Work out the finished part from the listing and answer in its coordinate system (mm). Face numbers are marked on the shaded views. A direction names the side the tool comes from. Give positions to 0.01 mm unless a question says otherwise; leave off trailing zeros. Order: outer loops, then holes, each group sorted by start corner. A loop starts at its lowest first (then second) coordinate and runs counter-clockwise, first axis right, second up.
```python
from build123d import *

# Parameters (mm, degrees)
EXTRUDE_1_DEPTH          = 2.5
SKETCH_5_R               = 0.6
CUT_EXTRUDE_1_DEPTH      = 19.036421485
CUT_EXTRUDE_START        = -2
SKETCH_5_3_R             = 1
CUT_EXTRUDE_2_DEPTH      = 1
REVOLVE_1_ANGLE          = 1
SKETCH_9_R               = 0.6
CUT_EXTRUDE_3_DEPTH      = 41.426698916
SKETCH_9_3_R             = 1
CUT_EXTRUDE_4_DEPTH      = 1
SKETCH_10_W              = 73.33326834
SKETCH_10_H              = 28.500223869
CUT_EXTRUDE_5_DEPTH      = 41.528606999
CUT_EXTRUDE_8_DEPTH      = 41.426698916
CUT_EXTRUDE_8_DEPTH_BACK = 41.426698916


with BuildPart() as part:
    # 草图4 → 凸台-拉伸1 (new body)
    with BuildSketch(Plane.XY):
        Polygon((8.5, -1.5), (17.75, -1.5), (17.75, -3.5), (-4.5, -3.5), (-4.5, -1.5), (-0.5, 0), (0, 0), (0, -1.5), (4, -1.5), (4, 0), (4.5, 0), align=None)
    extrude(amount=EXTRUDE_1_DEPTH)

    # 草图5 → 切除-拉伸1 (cut, through all)
    with BuildSketch(Plane(origin=(0, -1.5, 0), x_dir=(1, 0, 0), z_dir=(0, 1, 0))):
        with Locations(Location((2, -1.25, 0), (0, 0, 270))):
            Circle(SKETCH_5_R)
    extrude(amount=-CUT_EXTRUDE_1_DEPTH, mode=Mode.SUBTRACT)

    # 草图5<3> → 切除-拉伸2 (cut)
    with BuildSketch(Plane(origin=(0, -1.5, 0), x_dir=(1, 0, 0), z_dir=(0, 1, 0)).offset(CUT_EXTRUDE_START)):
        with Locations((2, -1.25)):
            Circle(SKETCH_5_3_R)
    extrude(amount=CUT_EXTRUDE_2_DEPTH, mode=Mode.SUBTRACT)

    # 镜向1: part across plane


with BuildPart() as part_1:
    add(part.part)
    add(part.part.mirror(Plane(origin=(17.75, 0, 2.5), x_dir=(0, 0, 1), z_dir=(1, 0, 0))))

    # 草图6 → 旋转1 (revolve)
    with BuildSketch(Plane.XY.offset(2.5)):
        Polygon((0, 0), (-0.5, 0), (-4.5, -1.5), (-4.5, -3.5), (40, -3.5), (40, -1.5), (36, 0), (35.5, 0), (35.5, -1.5), (31.5, -1.5), (31.5, 0), (31, 0), (27, -1.5), (8.5, -1.5), (4.5, 0), (4, 0), (4, -1.5), (0, -1.5), align=None)
    revolve(axis=Axis((-132.25, 94.8535776, 2.5), (0, -1, 0)), revolution_arc=REVOLVE_1_ANGLE)

    # 草图9 → 切除-拉伸3 (cut, through all)
    with BuildSketch(Plane(origin=(0, -1.5, 0), x_dir=(1, 0, 0), z_dir=(0, 1, 0))):
        with Locations(Location((1.994888171, -3.671537391, 0), (0, 0, 180))):
            Circle(SKETCH_9_R)
        with Locations(Location((33.493688748, -3.946423259, 0), (0, 0, 180))):
            Circle(SKETCH_9_R)
    extrude(amount=-CUT_EXTRUDE_3_DEPTH, mode=Mode.SUBTRACT)

    # 草图9<3> → 切除-拉伸4 (cut)
    with BuildSketch(Plane(origin=(0, -1.5, 0), x_dir=(1, 0, 0), z_dir=(0, 1, 0)).offset(CUT_EXTRUDE_START)):
        with Locations((1.994888171, -3.671537391)):
            Circle(SKETCH_9_3_R)
        with Locations((33.493688748, -3.946423259)):
            Circle(SKETCH_9_3_R)
    extrude(amount=CUT_EXTRUDE_4_DEPTH, mode=Mode.SUBTRACT)

    # 镜向2: part across plane


with BuildPart() as part_2:
    add(part_1.part)
    add(part_1.part.mirror(Plane.XY))

    # 草图10 → 切除-拉伸5 (cut, through all)
    with BuildSketch(Plane(origin=(0, 0, 0), x_dir=(-1, 0, 0), z_dir=(0, 0, -1))):
        with Locations((-19.859748979, -4.462825858)):
            Rectangle(SKETCH_10_W, SKETCH_10_H)
    extrude(amount=-CUT_EXTRUDE_5_DEPTH, mode=Mode.SUBTRACT)

    # 草图11 → 切除-拉伸8 (cut, two sides: drawn at the far end of the back side and taken through both)
    with BuildSketch(Plane(origin=(0, -1.5, 0), x_dir=(1, 0, 0), z_dir=(0, 1, 0)).offset(-CUT_EXTRUDE_8_DEPTH_BACK)):
        Polygon((8.5, 2.5), (8.5, 1.5), (11, 1.5), (9.834379916, 3.5), (14.665620084, 3.5), (13.5, 1.5), (18.331240168, 1.5), (17.165620084, 3.5), (21.996860252, 3.5), (20.831240168, 1.5), (25.662480335, 1.5), (24.496860252, 3.5), (26.996860252, 3.5), (27, 2.5), (40, 2.5), (40, 0), (-4.5, 0), (-4.5, 2.5), align=None)
    extrude(amount=CUT_EXTRUDE_8_DEPTH + CUT_EXTRUDE_8_DEPTH_BACK, mode=Mode.SUBTRACT)


solid = part_2.part
```
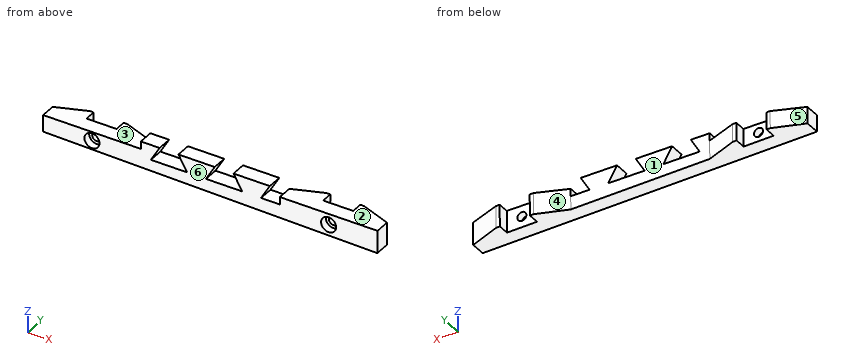
1. The mould has two halves that part along X. Classify the marked faces 4, 5 and 6: pulls with the +X half, pulls with the -X half, needs draft (parallel to the pull), parting line crosses it, or undercut.
Findings below:
face 4: undercut
face 5: pulls with the -X half
face 6: needs draft
2. The part is cut by section C-C (x = 0.5). Write down the section's boundary in (y, z).
Findings below:
outline: (-3.5, -4.82) - (-1.5, -4.82) - (-1.5, -2.5) - (-3.5, -2.5) - close
3. Which of the six approach directions +Z, -Z, +X, -X, +Y, -Y give full straight-line access (tool end or side, diameter ignored) to the marked faces 1, 2 and 3?
Findings below:
face 1: +Z, -Z, +Y
face 2: +Z, +X, +Y, -Y
face 3: +Z, -X, +Y, -Y
4. The part is cut by section A-A (y = -0.95). Write down the section's boundary in (x, z).
Findings below:
outline: (-3.05, -4.76) - (-0.02, -4.81) arc R132.25 ccw to (0, -2.5) - (-3.03, -2.5) arc R129.22 cw to start; (3.98, -4.88) - (7.01, -4.93) arc R139.28 ccw to (7.03, -2.5) - (4, -2.5) arc R136.25 cw to start; (28.44, -5.3) - (31.48, -5.36) arc R163.75 ccw to (31.5, -2.5) - (28.47, -2.5) arc R160.72 cw to start; (35.47, -5.43) - (38.51, -5.48) arc R170.78 ccw to (38.53, -2.5) - (35.5, -2.5) arc R167.75 cw to start
5. The part is cut by section B-B (x = 32). Write down the section's boundary in (y, z), then the cut area to 3 significant figures.
Findings below:
outline: (-3.5, -5.37) - (-1.5, -5.37) - (-1.5, -2.5) - (-3.5, -2.5) - close
area: 5.73 mm2
6. Given P1, Ø0.7, axis at x = 3, z = -4, coming from the +Y side; P2, Ø1.8, axis at x = 1, y = -2, coming from the +Z side; P3, Ø1.8, axis at x = 1.99, z = -3.67, coming from the -Y side, each flat-ended and moving along its own axis, determine where each tip first touches the part or whether it passes through.
Findings below:
P1: stops at y = -1.5
P2: stops at z = -2.5
P3: stops at y = -2.5
7. Straight lines are drawn through the part: probe 1 along X at (y, z) = (-2.3, -3.85); probe 2 along X at (y, z) = (-2.15, -2.7); probe 3 along X at (y, z) = (-2.2, -2.9). For each, find the intervals that lie inside material, in ascending order.
Findings below:
probe 1: x = -4.51 to 1.42, 2.57 to 32.9, 34.09 to 39.99
probe 2: x = -4.5 to 10.3, 14.2 to 17.63, 21.53 to 24.96, 27 to 40
probe 3: x = -4.5 to 10.18, 14.32 to 17.52, 21.65 to 24.85, 27 to 40
